Geometry: final body of the model. Coordinates: model frame, mm. Face numbers are marked on the shaded views. A direction names the side the tool comes from. Round coordinates to 2 decimals unless told otherwise and drop trailing zeros. Loops run counter-clockwise (first coordinate to the right, second up) from the corner with the lowest first, then second, coordinate; pieces in that order, holes last. Notation, with made-up numbers: (-12, -35) -> (20, -35) arc R27 cw to (20, -8) -> close; hole circle Ø8 at (63.25, 22.5). An arc over 180 degrees is marked (long way). Answer in a Markdown table with one row per item.
```python
from build123d import *
from OCP.BRepFilletAPI import BRepFilletAPI_MakeFillet

# Parameters (mm, degrees)
SKETCH1_W           = 5.5
SKETCH1_H           = 5.5
BOSS_EXTRUDE1_DEPTH = 1.5
SKETCH5_W           = 5
SKETCH5_H           = 5
BOSS_EXTRUDE2_DEPTH = 3
SKETCH2_W           = 3.5
SKETCH2_H           = 3.5
CUT_EXTRUDE1_DEPTH  = 2
SKETCH10_W          = 3.5
SKETCH10_H          = 1.5
CUT_EXTRUDE3_DEPTH  = 9.031189202
FILLET7_R1          = 0.5
FILLET7_R2          = 1.5
BOSS_EXTRUDE3_DEPTH = 1.5


with BuildPart() as part:
    # Sketch1 → Boss-Extrude1 (new, symmetric)
    with BuildSketch(Plane.XY):
        with Locations((2.75, 2.75)):
            Rectangle(SKETCH1_W, SKETCH1_H)
        with Locations((-2.75, 2.75)):
            Rectangle(SKETCH1_W, SKETCH1_H)
    extrude(amount=BOSS_EXTRUDE1_DEPTH, both=True)

    # Sketch5 → Boss-Extrude2 (add)
    with BuildSketch(Plane.XY.offset(1.5)):
        with Locations((0, -2.5)):
            Rectangle(SKETCH5_W, SKETCH5_H)
    extrude(amount=-BOSS_EXTRUDE2_DEPTH)

    # Sketch2 → Cut-Extrude1 (cut)
    with BuildSketch(Plane.XY.offset(1.5)):
        with Locations((2.75, 2.75)):
            Rectangle(SKETCH2_W, SKETCH2_H)
        with Locations((-2.75, 2.75)):
            Rectangle(SKETCH2_W, SKETCH2_H)
        with Locations((0, -2.5)):
            Rectangle(SKETCH2_W, SKETCH2_H)
    extrude(amount=-CUT_EXTRUDE1_DEPTH, mode=Mode.SUBTRACT)

    # Sketch10 → Cut-Extrude3 (cut, through all)
    with BuildSketch(Plane.XY.offset(-0.5)):
        with Locations((0, -2.5)):
            Rectangle(SKETCH10_W, SKETCH10_H)
        with Locations((2.75, 2.75)):
            Rectangle(SKETCH10_W, SKETCH10_H)
        with Locations((-2.75, 2.75)):
            Rectangle(SKETCH10_W, SKETCH10_H)
    extrude(amount=-CUT_EXTRUDE3_DEPTH, mode=Mode.SUBTRACT)

    # Fillet7: one fillet with a radius per group of edges: ONE call of the kernel's fillet builder (fillet() takes one radius for all edges)
    fillet7_edges_1 = [part.edges().sort_by_distance(p)[0] for p in [
        (5.5, 0, 0),
        (2.5, -5, 0),
        (5.5, 5.5, 0),
        (-5.5, 5.5, 0),
        (-5.5, 0, 0),
        (-2.5, -5, 0),
    ]]
    fillet7_edges_2 = [part.edges().sort_by_distance(p)[0] for p in [
        (2.5, 0, 0),
        (-2.5, 0, 0),
    ]]
    fillet7 = BRepFilletAPI_MakeFillet(part.part.solid().wrapped)
    for e in fillet7_edges_1:
        fillet7.Add(FILLET7_R1, e.wrapped)
    for e in fillet7_edges_2:
        fillet7.Add(FILLET7_R2, e.wrapped)
    add(Compound.cast(fillet7.Shape()), mode=Mode.REPLACE)

    # Sketch11 → Boss-Extrude3 (add, through all)
    with BuildSketch(Plane.XY):
        with BuildLine():
            ThreePointArc((-6.301018176, -11.939311954), (8.8396e-05, -13.5), (6.301174529, -11.939229437))
            ThreePointArc((6.301174529, -11.939229437), (6.554033768, -9.398401396), (4.941977619, -7.41824486))
            ThreePointArc((4.941977619, -7.41824486), (4.139435534, -3.238722534), (8.395134632, -3.277528018))
            ThreePointArc((8.395134632, -3.277528018), (10.526696598, -4.494141765), (12.915304874, -3.93))
            ThreePointArc((12.915304874, -3.93), (11.870145687, 6.430368681), (3.762845966, 12.964990946))
            ThreePointArc((3.762845966, 12.964990946), (2.804609837, 11.521965342), (2.695822199, 9.793178304))
            ThreePointArc((2.695822199, 9.793178304), (0, 6.5), (-2.695822199, 9.793178304))
            ThreePointArc((-2.695822199, 9.793178304), (-2.804609837, 11.521965342), (-3.762845966, 12.964990946))
            ThreePointArc((-3.762845966, 12.964990946), (-11.870183671, 6.430298564), (-12.915258444, -3.930152581))
            ThreePointArc((-12.915258444, -3.930152581), (-10.526666364, -4.494205663), (-8.395162612, -3.277562841))
            ThreePointArc((-8.395162612, -3.277562841), (-4.139464145, -3.238688227), (-4.941938337, -7.418223589))
            ThreePointArc((-4.941938337, -7.418223589), (-6.553975653, -9.398450665), (-6.301018176, -11.939311954))
        make_face()
        with BuildLine():
            Line((-2.5, -1.5), (-2.5, -4.5))
            ThreePointArc((-2.5, -4.5), (-2.353553391, -4.853553391), (-2, -5))
            Line((-2, -5), (2, -5))
            ThreePointArc((2, -5), (2.353553391, -4.853553391), (2.5, -4.5))
            Line((2.5, -4.5), (2.5, -1.5))
            ThreePointArc((2.5, -1.5), (2.939339828, -0.439339828), (4, 0))
            Line((4, 0), (5, 0))
            ThreePointArc((5, 0), (5.353553391, 0.146446609), (5.5, 0.5))
            Line((5.5, 0.5), (5.5, 5))
            ThreePointArc((5.5, 5), (5.353553391, 5.353553391), (5, 5.5))
            Line((5, 5.5), (-5, 5.5))
            ThreePointArc((-5, 5.5), (-5.353553391, 5.353553391), (-5.5, 5))
            Line((-5.5, 5), (-5.5, 0.5))
            ThreePointArc((-5.5, 0.5), (-5.353553391, 0.146446609), (-5, 0))
            Line((-5, 0), (-4, 0))
            ThreePointArc((-4, 0), (-2.939339828, -0.439339828), (-2.5, -1.5))
        make_face(mode=Mode.SUBTRACT)
    extrude(amount=-BOSS_EXTRUDE3_DEPTH)


solid = part.part
```
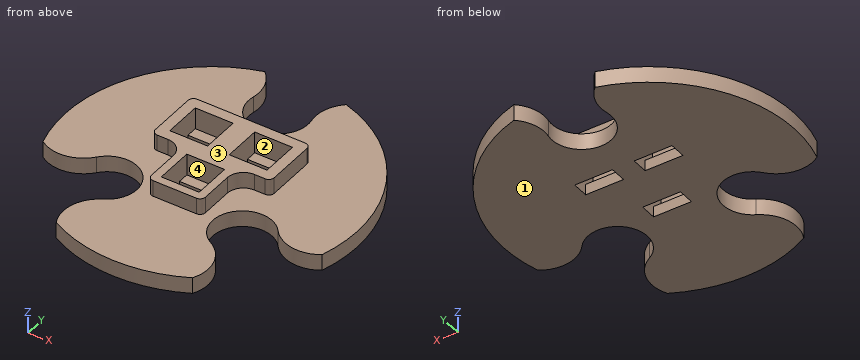
Item 1: Draft query along Y for the marked faces 1 and 2. Return one class per face: pulls with the +Y half, pulls with the -Y half, needs draft (parallel to the pull), parting line crosses it, or undercut.
Answer:
| item | result |
|---|---|
| face 1 | needs draft |
| face 2 | undercut |
Item 2: Line query: probe 1 along X at (y, z) = (1.75, 0.15); probe 2 along Y at (x, z) = (4.25, -0.85); probe 3 along Y at (x, z) = (0, -1.15). Output: solid intervals per line, ascending. Write a range as [from, to].
Answer:
| item | result |
|---|---|
| probe 1 | x = [-5.5, -4.5], [-1, 1], [4.5, 5.5] |
| probe 2 | y = [-12.81, -6.89], [-3.11, 2], [3.5, 12.81] |
| probe 3 | y = [-13.5, -3.25], [-1.75, 6.5] |
Item 3: Cut plane D-D (y = -8). Output: boundary loops of the cut face in (x, z).
Answer:
| item | result |
|---|---|
| outline | (-5.72, -1.5) -> (5.72, -1.5) -> (5.72, 0) -> (-5.72, 0) -> close |
Item 4: Cut plane C-C (y = 9). Output: boundary loops of the cut face in (x, z), then the cut area to 3 significant figures.
Answer:
| item | result |
|---|---|
| outline | (-10.06, -1.5) -> (-2.74, -1.5) -> (-2.74, 0) -> (-10.06, 0) -> close; (2.74, -1.5) -> (10.06, -1.5) -> (10.06, 0) -> (2.74, 0) -> close |
| area | 22.0 mm² |
Item 5: Cut plane A-A (x = 0). Output: boundary loops of the cut face in (y, z).
Answer:
| item | result |
|---|---|
| outline | (-13.5, -1.5) -> (-3.25, -1.5) -> (-3.25, -0.5) -> (-4.25, -0.5) -> (-4.25, 1.5) -> (-5, 1.5) -> (-5, 0) -> (-13.5, 0) -> close; (-1.75, -1.5) -> (6.5, -1.5) -> (6.5, 0) -> (5.5, 0) -> (5.5, 1.5) -> (-0.75, 1.5) -> (-0.75, -0.5) -> (-1.75, -0.5) -> close |
Item 6: Cut plane B-B (z = 0.6). Output: boundary loops of the cut face in (x, y), then the cut area to 3 significant figures.
Answer:
| item | result |
|---|---|
| outline | (-5.5, 0.5) arc R0.5 ccw to (-5, 0) -> (-4, 0) arc R1.5 cw to (-2.5, -1.5) -> (-2.5, -4.5) arc R0.5 ccw to (-2, -5) -> (2, -5) arc R0.5 ccw to (2.5, -4.5) -> (2.5, -1.5) arc R1.5 cw to (4, 0) -> (5, 0) arc R0.5 ccw to (5.5, 0.5) -> (5.5, 5) arc R0.5 ccw to (5, 5.5) -> (-5, 5.5) arc R0.5 ccw to (-5.5, 5) -> close; hole (-4.5, 1) -> (-1, 1) -> (-1, 4.5) -> (-4.5, 4.5) -> close; hole (-1.75, -4.25) -> (1.75, -4.25) -> (1.75, -0.75) -> (-1.75, -0.75) -> close; hole (1, 1) -> (4.5, 1) -> (4.5, 4.5) -> (1, 4.5) -> close |
| area | 49.4 mm² |
Item 7: Pin query (flat end, axial travel): pin 1 Ø0.8 at (x, z) = (0.5, 1) entering from -Y; pin 2 Ø0.5 at (x, z) = (-4.5, 0.5) entering from -Y; pin 3 Ø0.6 at (x, z) = (3, 0) entering from +Y. Return the tip coordinate at first contact, or that it passes through.
Answer:
| item | result |
|---|---|
| pin 1 | stops at y = -5 |
| pin 2 | stops at y = 0 |
| pin 3 | stops at y = 12.46 |
Item 8: Reachability of the marked faces 3 and 4 from +Z, -Z, +X, -X, +Y, -Y: full face, straight path, thin tool, end or side. Return the list, or none.
Answer:
| item | result |
|---|---|
| face 3 | +Z, +X, -X, +Y, -Y |
| face 4 | +Z |
